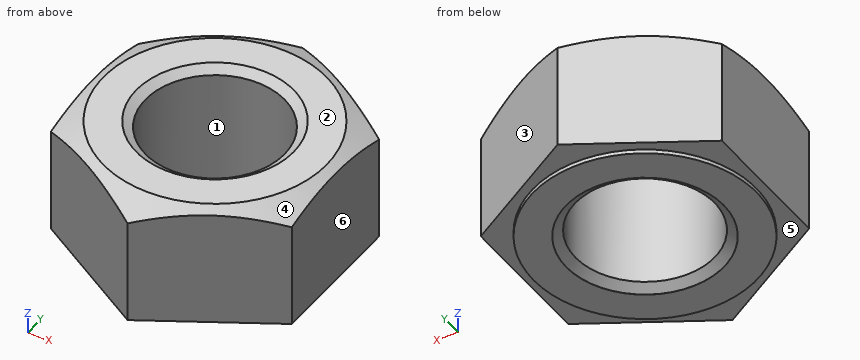
from build123d import *

# Parameters (mm, degrees)
BASENUT_START = -24
BASENUTSKE_R  = 13.25
BASENUT_DEPTH = 24
SKETCH4_W     = 0.8
SKETCH4_H     = 15.308112383


# Read off the part's stored shape, not the designer's step: ThreadSchematic
with BuildPart() as part:
    # BaseNutSke → BaseNut (new body)
    with BuildSketch(Plane.XY.offset(BASENUT_START)):
        Polygon((23, 13.279056191), (23, -13.279056191), (0, -26.558112383), (-23, -13.279056191), (-23, 13.279056191), (0, 26.558112383), align=None)
        Circle(BASENUTSKE_R, mode=Mode.SUBTRACT)
    extrude(amount=BASENUT_DEPTH)

    # Sketch5 (on Front Plane) → EndChamfer (revolve, cut)
    with BuildSketch(Plane.XY):
        Polygon((23.9746, 15), (22.626700489, 13.075), (24.0254, 13.075), (24.0254, 15), align=None)
    revolve(axis=Axis((23.9746, 15, 0), (-0.5735764363510466, -0.8191520442889915, 0)), mode=Mode.SUBTRACT)

    # Sketch4 → Bearing-Face (revolve, cut)
    with BuildSketch(Plane(origin=(0, 0, 0), x_dir=(0, 0, -1), z_dir=(1, 0, 0)), mode=Mode.PRIVATE) as bearing_face_sk:
        with Locations((23.6, 28.904056192)):
            Rectangle(SKETCH4_W, SKETCH4_H)
        Polygon((0, 21.25), (-10, 21.25), (-10, 36.558112383), (3.064640113, 36.558112383), (3.064640113, 26.558112383), align=None)
    revolve(bearing_face_sk.sketch.rotate(Axis((0, 0, 0), (0, 0, -1)), 90), axis=Axis((0, 0, 0), (0, 0, -1)), mode=Mode.SUBTRACT)

    # ThreadSchematic outline → ThreadSchematic (revolve, cut)
    with BuildSketch(Plane.XZ):
        Polygon((13.25, 0), (13.25, -1.225363192), (15, 0), align=None)
        Polygon((15, -23.9746), (13.25, -22.749236808), (13.25, -24), (15, -24), align=None)
    revolve(axis=Axis((0, 0, 0), (0, 0, 1)), mode=Mode.SUBTRACT)


solid = part.part
The listing builds one solid part. Answer for the finished solid, in the listing's coordinates (mm). Face numbers are marked on the shaded views. A direction names the side the tool comes from. Give positions to 0.01 mm unless a question says otherwise; leave off trailing zeros. Write each loop counter-clockwise with the first axis right and the second up, starting at its lowest first coordinate (ties: lowest second). Pieces come first, ordered by that corner, then holes.
1) A tool of negligible diameter and unlimited length cuts with its end or side. For the marked faces 5 and 6, from which of +Z, -Z, +X, -X, +Y, -Y can it reach the whole face along a straight path? Write none if from no direction.
2) Section B-B (z = -16.5) is taken. Write down the section's boundary in (x, y).
3) Given P1, Ø16, axis at x = 0, y = 0, coming from the -Z side; P2, Ø2, axis at x = 13, z = -20.5, coming from the -Y side; P3, Ø3, axis at x = 11, y = 20.5, coming from the +Z side; P4, Ø5, axis at x = -17, z = -12, coming from the -Y side, each flat-ended and moving along its own axis, determine where each tip first touches the part or whether it passes through.
4) For a pull along X with two mould halves and no side action, classify the marked faces 1, 2, 3 and 4 as pulls with the +X half, pulls with the -X half, needs draft (parallel to the pull), parting line crosses it, or undercut.
5) Find the intervals of material crossed by L1, parallel to Y at x = -20, z = -11.75; L2, parallel to Y at x = -10.5, z = -4.5; L3, parallel to Y at x = 0, z = -7, in increasing order.
Response:
1. face 5: -Z
1. face 6: +Z, -Z, +X, +Y, -Y
2. outline: (-23, -13.28) - (0, -26.56) - (23, -13.28) - (23, 13.28) - (0, 26.56) - (-23, 13.28) - close; hole circle Ø26.5 at (0, 0)
3. P1: passes through
3. P2: stops at y = -19.63
3. P3: stops at z = -0.3
3. P4: stops at y = -18.19
4. face 1: undercut
4. face 2: needs draft
4. face 3: pulls with the +X half
4. face 4: parting line crosses it
5. L1: y = -15.01 to 15.01
5. L2: y = -20.5 to -8.08, 8.08 to 20.5
5. L3: y = -26.56 to -13.25, 13.25 to 26.56
